Geometry check sheet. Reference: the model listing, model coordinates, mm. A direction names the side the tool comes from. Coordinates: 2 decimals unless noted, no trailing zeros. Loops run counter-clockwise (first coordinate to the right, second up) from the corner with the lowest first, then second, coordinate; pieces in that order, holes last.
from build123d import *

# Parameters (mm, degrees)
SKETCH1_R           = 30
BOSS_EXTRUDE1_DEPTH = 30


with BuildPart() as part:
    # Sketch1 → Boss-Extrude1 (new body)
    with BuildSketch(Plane.XY):
        with BuildLine():
            Line((-163.480061578, 42.114452454), (-291.506249588, 38.739141102))
            ThreePointArc((-291.506249588, 38.739141102), (-373.11762328, 0), (-291.506249588, -38.739141102))
            Line((-291.506249588, -38.739141102), (-161.55881164, -42.158253128))
            Line((-161.55881164, -42.158253128), (163.480061578, -42.158253128))
            Line((163.480061578, -42.158253128), (283.79954089, -30.888321372))
            ThreePointArc((283.79954089, -30.888321372), (373.11762328, 0), (283.79954089, 30.888321372))
            Line((283.79954089, 30.888321372), (163.480061578, 42.114452454))
            Line((163.480061578, 42.114452454), (-163.480061578, 42.114452454))
        make_face()
        with Locations((-323.11762328, 0)):
            Circle(SKETCH1_R, mode=Mode.SUBTRACT)
        with Locations((323.11762328, 0)):
            Circle(SKETCH1_R, mode=Mode.SUBTRACT)
    extrude(amount=BOSS_EXTRUDE1_DEPTH)


solid = part.part
(1) Scan lines: L1, parallel to X at y = -8, z = 26.25; L2, parallel to X at y = 16, z = 12; L3, parallel to Y at x = -321, z = 18.5. Record each from-to range of solid material in increasing order.
Findings:
L1: x = -372.47 to -352.03, -294.2 to 294.2, 352.03 to 372.47
L2: x = -370.49 to -348.49, -297.74 to 297.74, 348.49 to 370.49
L3: y = -49.96 to -29.93, 29.93 to 49.96
(2) Gauge pin test, flat ends, axial feed: pin 1 Ø10 at (x, z) = (50, 5) entering from -Y; pin 2 Ø4 at (y, z) = (38, 22) entering from +X; pin 3 Ø1 at (y, z) = (-18.5, 16) entering from +X. Record the tip position at first contact, or that the pin passes through.
Findings:
pin 1: stops at y = -42.16
pin 2: stops at x = 357.82
pin 3: stops at x = 369.77
(3) Access from +Z, -Z, +X, -X, +Y, -Y to the whole of each face (thin tool, end or side, straight path). Record for faces 4 (the flat face through (-5, 1, 30)), 5 (the flat face through (-1, -42.158, 15)), 6 (the flat face through (2, 42.114, 15)).
Findings:
face 4: +Z, +X, -X, +Y, -Y
face 5: +Z, -Z, -Y
face 6: +Z, -Z, +Y
(4) Sectioned sample at C-C on x = -41. Record the cut outline in (y, z).
Findings:
outline: (-42.16, 0) - (42.11, 0) - (42.11, 30) - (-42.16, 30) - close
(5) Sectioned sample at A-A on y = 0. Record the cut outline in (x, z).
Findings:
outline: (-373.12, 0) - (-353.12, 0) - (-353.12, 30) - (-373.12, 30) - close; (-293.12, 0) - (293.12, 0) - (293.12, 30) - (-293.12, 30) - close; (353.12, 0) - (373.12, 0) - (373.12, 30) - (353.12, 30) - close
(6) Sectioned sample at B-B on z = 24.75. Record the cut outline in (x, y).
Findings:
outline: (-291.51, -38.74) - (-161.56, -42.16) - (163.48, -42.16) - (283.8, -30.89) arc R50 ccw (long way) to (283.8, 30.89) - (163.48, 42.11) - (-163.48, 42.11) - (-291.51, 38.74) arc R50 ccw (long way) to start; hole circle Ø60 at (-323.12, 0); hole circle Ø60 at (323.12, 0)
(7) Draft check along Y on faces 1 (the cylindrical face through (-294.5, 9, 14.8)), 2 (the cylindrical face through (373.088, -1.733, 14.79)), 3 (the flat face through (-5, 1, 0)). Enter one of: +Y half, -Y half, draft (parallel to the pull), parting line (faces both ways), or undercut.
Findings:
face 1: undercut
face 2: parting line
face 3: draft
